Here's how the part is built. I have some questions about the finished solid (model axes, mm). A direction names the side the tool comes from. Coordinates: 2 decimals unless noted, no trailing zeros. Order: outer loops, then holes, each group sorted by start corner. A loop starts at its lowest first (then second) coordinate and runs counter-clockwise, first axis right, second up. Notation, with made-up numbers: (60.5, 47.25) - (83.5, 47.25) arc R31 ccw to (83.5, 84.25) - close; hole circle Ø2 at (66, -38). An arc over 180 degrees is marked (long way). Answer in a Markdown table with one row per item. Add a question column.
Item 1: Will these pins go through, and if not, where does the flat tip stop? pin 1 Ø1.5 at (x, y) = (-16, -5) entering from +Z; pin 2 Ø2 at (x, z) = (16, 3.5) entering from -Y; pin 3 Ø12 at (x, y) = (14, -12) entering from +Z; pin 4 Ø12 at (x, y) = (3, -5.5) entering from +Z.
Item 2: I want a section at D-D (z = 8). Please give me the cut outline in (x, y), plus the area to 3 significant figures.
Item 3: Thinking about a two-plate mould opening in X: for faces 1 (the cylindrical face through (-6.33, -5.63, -10.97)), 2 (the cylindrical face through (-13.205, -5.635, -0.791)), 3 (the flat face through (4, 0, 0)), which applies, +X half, -X half, draft (parallel to the pull), parting line (faces both ways), or undercut?
Item 4: I want a section at B-B (x = 0). Please give me the cut outline in (y, z).
Item 5: On a 3-axis mill with a long thin cutter (end or side, diameter ignored), from which of +Z, -Z, +X, -X, +Y, -Y can I reach the whole of each face in a straight line? I mean faces 4 (the cylindrical face through (-19.679, -5.635, -3.745)), 5 (the cylindrical face through (-5.029, -30.188, -3.856)). Say none if no direction works.
Item 6: I want a section at C-C (y = -34). Please give me the cut outline in (x, z).
Item 7: If I drill on line 1 along Y through (x, z) = (-7.5, -6.5); line 2 along Y through (x, z) = (3.5, -6); line 3 along X through (y, z) = (-13.5, -3), over which ranges is the centre line in solid material (lowest first)? Write a range as from..to.
Item 8: I want a section at A-A (y = -8). Please give me the cut outline in (x, z).
```python
from build123d import *

# Parameters (mm, degrees)
F0_R     = 2.065749
F0_R_2   = 6.9977
F1_DEPTH = 11.43
F0_R_3   = 6.3373
F2_DEPTH = 23.0124
F3_DEPTH = 37.5666


with BuildPart() as f1:
    # F0 (on Front) → F1 (new body)
    with BuildSketch(Plane.XZ):
        with BuildLine():
            ThreePointArc((-14.886502, -5.901155), (-6.237069, -11.087668), (-3.319826, -20.741803))
            ThreePointArc((-3.319826, -20.741803), (21.0058, 0), (-3.319826, 20.741803))
            ThreePointArc((-3.319826, 20.741803), (-6.237069, 11.087668), (-14.886502, 5.901155))
            ThreePointArc((-14.886502, 5.901155), (-15.747764, 5.779367), (-16.614929, 5.711317))
            ThreePointArc((-16.614929, 5.711317), (-19.646861, 3.78405), (-21.000843, 0.456331))
            ThreePointArc((-21.000843, 0.456331), (-21.0058, 0), (-21.000843, -0.456331))
            ThreePointArc((-21.000843, -0.456331), (-19.646861, -3.78405), (-16.614929, -5.711317))
            ThreePointArc((-16.614929, -5.711317), (-15.747764, -5.779367), (-14.886502, -5.901155))
        make_face()
        with Locations((-15.113, 0)):
            Circle(F0_R, mode=Mode.SUBTRACT)
        Circle(F0_R_2, mode=Mode.SUBTRACT)
        with BuildLine():
            ThreePointArc((-16.614929, -5.711317), (-15.757741, -5.870199), (-14.886502, -5.901155))
            ThreePointArc((-14.886502, -5.901155), (-15.747764, -5.779367), (-16.614929, -5.711317))
        make_face()
        with BuildLine():
            ThreePointArc((-16.614929, 5.711317), (-15.747764, 5.779367), (-14.886502, 5.901155))
            ThreePointArc((-14.886502, 5.901155), (-15.757741, 5.870199), (-16.614929, 5.711317))
        make_face()
        with BuildLine():
            ThreePointArc((-21.000843, 0.456331), (-21.0185, 0), (-21.000843, -0.456331))
            ThreePointArc((-21.000843, -0.456331), (-21.0058, 0), (-21.000843, 0.456331))
        make_face()
    extrude(amount=F1_DEPTH)

    # F0 (on Front) → F2 (join)
    with BuildSketch(Plane.XZ):
        Circle(F0_R_2)
        Circle(F0_R_3, mode=Mode.SUBTRACT)
    extrude(amount=F2_DEPTH)

    # F0 (on Front) → F3 (join)
    with BuildSketch(Plane.XZ):
        Circle(F0_R_3)
    extrude(amount=F3_DEPTH)


solid = f1.part
```
Values follow:
| question | item | result |
|---|---|---|
| 1 | pin 1 | stops at z = 5.9 |
| 1 | pin 2 | stops at y = -11.43 |
| 1 | pin 3 | stops at z = 19.41 |
| 1 | pin 4 | stops at z = 21.01 |
| 2 | outline | (-9.58, -11.43) - (19.42, -11.43) - (19.42, 0) - (-9.58, 0) - close |
| 2 | area | 332 mm^2 |
| 3 | face 1 | -X half |
| 3 | face 2 | undercut |
| 3 | face 3 | draft |
| 4 | outline | (-37.57, -6.34) - (-23.01, -6.34) - (-23.01, -7) - (-11.43, -7) - (-11.43, -21.01) - (0, -21.01) - (0, 21.01) - (-11.43, 21.01) - (-11.43, 7) - (-23.01, 7) - (-23.01, 6.34) - (-37.57, 6.34) - close |
| 5 | face 4 | -Z, -X, +Y, -Y |
| 5 | face 5 | -Y |
| 6 | outline | circle Ø12.67 at (0, 0) |
| 7 | line 1 | y = -11.43..0 |
| 7 | line 2 | y = -23.01..0 |
| 7 | line 3 | x = -6.32..6.32 |
| 8 | outline | (-21, -0.46) arc R5.91 ccw to (-16.61, -5.71) arc R5.91 ccw to (-14.89, -5.9) arc R14 cw to (-3.32, -20.74) arc R21.01 ccw (long way) to (-3.32, 20.74) arc R14 cw to (-14.89, 5.9) arc R5.91 ccw to (-16.61, 5.71) arc R5.91 ccw to (-21, 0.46) arc R5.91 ccw to start; hole circle Ø4.13 at (-15.11, 0) |
